Source: three-view drawing plus pictorial views. Frame: mm from the lowest corner of the part. Round coordinates to 2 decimals unless told otherwise and drop trailing zeros. Loops run counter-clockwise (first coordinate to the right, second up) from the corner with the lowest first, then second, coordinate; pieces in that order, holes last. Notation, with made-up numbers: M 17,47 L 48,47 A27 ccw 48,77 Z; hole C 75,84 d9. An arc over 180 degrees is marked long. Answer as a JSON object with one key per item and string values.
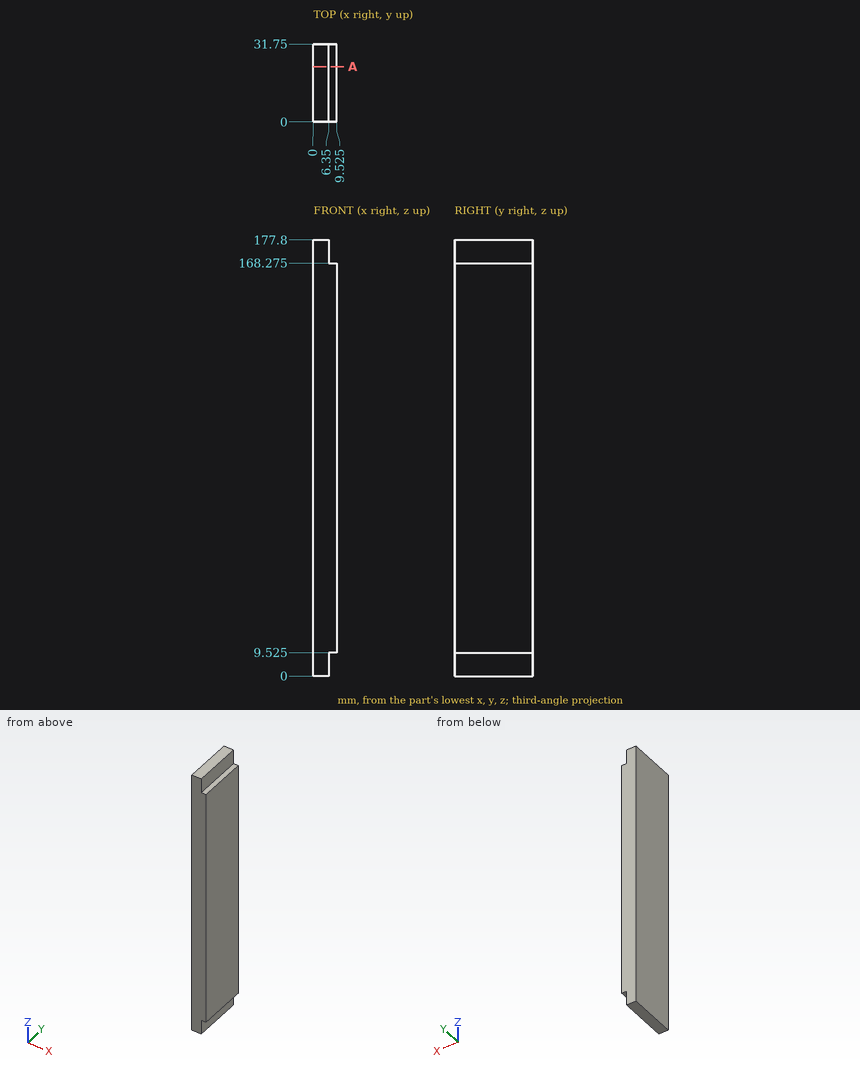
1) Line query: probe 1 along Z at (x, y) = (8.75, 22) (3 decimals); probe 2 along X at (y, z) = (10, 169.5). Output: solid intervals per line, ascending.
Geometry results:
{"probe 1": "9.525 to 168.275", "probe 2": "0 to 6.35"}
2) First-contact query: pin 1 (3 mm diameter, centred on x = 7, z = 80, fed in from -Y); pin 2 (10.5 mm diameter, centred on y = 23.5, z = 3.5, fed in from +X); pin 3 (1 mm diameter, centred on x = 8.5, y = 22, fed in from +Z) (3 decimals); pin 4 (1 mm diameter, centred on x = 7.5, y = 20, fed in from -Z) (3 decimals). Flat tips, straight axial feed; report the tip coordinate or a pass-through.
Geometry results:
{"pin 1": "y = 0", "pin 2": "x = 6.35", "pin 3": "z = 168.275", "pin 4": "z = 9.525"}
3) Cut plane A-A on y = 22.5. Return the cut outline in (x, z) (3 decimals), and give its area (3 significant figures).
Geometry results:
{"outline": "M 0,0 L 6.35,0 L 6.35,9.525 L 9.525,9.525 L 9.525,168.275 L 6.35,168.275 L 6.35,177.8 L 0,177.8 Z", "area": "1,630 mm2"}
